```python
from build123d import *

# Parameters (mm, degrees)
CROQUIS1_R                   = 5.25
SALIENTE_EXTRUIR1_DEPTH      = 10
CROQUIS2_R                   = 3
CORTAR_EXTRUIR1_DEPTH        = 10
SALIENTE_EXTRUIR2_DEPTH      = 2
SALIENTE_EXTRUIR2_DEPTH_BACK = 10
CROQUIS3_R                   = 1.25
REDONDEO1_R                  = 1.25


with BuildPart() as part:
    # Croquis1 → Saliente-Extruir1 (new body)
    with BuildSketch(Plane(origin=(0, 0, 0), x_dir=(1, 0, 0), z_dir=(0, 1, 0))):
        with Locations(Location((0, 0, 0), (0, 0, 270))):
            Circle(CROQUIS1_R)
    extrude(amount=SALIENTE_EXTRUIR1_DEPTH)

    # Croquis2 → Cortar-Extruir1 (cut)
    with BuildSketch(Plane(origin=(0, 10, 0), x_dir=(1, 0, 0), z_dir=(0, 1, 0))):
        with Locations(Location((0, 0, 0), (0, 0, 270))):
            Circle(CROQUIS2_R)
    extrude(amount=-CORTAR_EXTRUIR1_DEPTH, mode=Mode.SUBTRACT)

    # Croquis3 → Saliente-Extruir2 (add, two sides: drawn at the far end of the back side and taken through both)
    with BuildSketch(Plane(origin=(0, 10, 0), x_dir=(1, 0, 0), z_dir=(0, 1, 0)).offset(-SALIENTE_EXTRUIR2_DEPTH_BACK)):
        with Locations(Location((0, 3, 0), (0, 0, 270))):
            Circle(CROQUIS3_R)
        with Locations(Location((2.599576211, -1.499133975, 0), (0, 0, 270))):
            Circle(CROQUIS3_R)
        with Locations(Location((-2.596576211, -1.500866025, 0), (0, 0, 270))):
            Circle(CROQUIS3_R)
    extrude(amount=SALIENTE_EXTRUIR2_DEPTH + SALIENTE_EXTRUIR2_DEPTH_BACK)

    # Redondeo1
    redondeo1_edges = [part.edges().sort_by_distance(p)[0] for p in [
        (0, 12, -4.25),
        (2.599576211, 12, 0.249133975),
        (-2.596576211, 12, 0.250866025),
    ]]
    fillet(redondeo1_edges, radius=REDONDEO1_R)


solid = part.part
```
The model under review builds one solid part; all positions refer to its coordinate system, in mm. Round coordinates to 2 decimals unless told otherwise and drop trailing zeros. Loops run counter-clockwise (first coordinate to the right, second up) from the corner with the lowest first, then second, coordinate; pieces in that order, holes last. Notation, with made-up numbers: (11, -34) - (42, -34) arc R28 ccw to (42, -5) - close; hole circle Ø11 at (-20.75, -27). An arc over 180 degrees is marked (long way). Use a Markdown table: item, result. Add a question column.
Q1. Insertion check: pin 1 Ø2 at (x, y) = (4, 4.5) entering from +Z; pin 2 Ø2 at (y, z) = (10, 2) entering from +X; pin 3 Ø4 at (y, z) = (5.5, -4) entering from -X. Each pin has a flat end and moves straight along its axis. Give the tip position at first contact, or say it passes through.
Q2. Add section A-A (x = 0). State the section outline as (y, z) points.
Q3. The part is to be moulded in two halves that separate along Z. For faces 1 (the face through (-2.6, 5.1, -1.5)), 2 (the face through (-2, 0, 1)), 3 (the face through (1.6, 4.9, 5)), say which applies: pulls with the +Z half, pulls with the -Z half, needs draft (parallel to the pull), parting line crosses it, or undercut.
Q4. For probe 1 along Z at (x, y) = (-1.5, 1.25); probe 2 along Y at (x, z) = (3.5, 3.25); probe 3 along X at (y, z) = (8.25, -2), list the stretches that pass through material, from the lowest coordinate up.
Q5. Add section D-D (x = -1.5). State the section outline as (y, z) points, plus the area to 3 significant figures.
Q6. Add section B-B (z = 0). State the section outline as (x, y) points, plus the area to 3 significant figures.
Q7. Add section C-C (y = 6.75). State the section outline as (x, z) points.
Worked answers:
| question | item | result |
|---|---|---|
| 1 | pin 1 | z = 4.31 |
| 1 | pin 2 | x = 5.15 |
| 1 | pin 3 | x = -4.85 |
| 2 | outline | (0, -5.25) - (10, -5.25) - (10, -4.25) - (10.75, -4.25) arc R1.25 ccw to (10.75, -1.75) - (0, -1.75) - close; (0, 3) - (10, 3) - (10, 5.25) - (0, 5.25) - close |
| 3 | face 1 | undercut |
| 3 | face 2 | needs draft |
| 3 | face 3 | parting line crosses it |
| 4 | probe 1 | -5.03 to -2.6, 0.9 to 2.1, 2.6 to 5.03 |
| 4 | probe 2 | 0 to 10 |
| 4 | probe 3 | -4.85 to -2.24, -0.75 to 0.75, 2.24 to 4.85 |
| 5 | outline | (0, -5.03) - (10, -5.03) - (10, -2.6) - (0, -2.6) - close; (0, 0.9) - (10.75, 0.9) arc R0.6 ccw to (10.75, 2.1) - (0, 2.1) - close; (0, 2.6) - (10, 2.6) - (10, 5.03) - (0, 5.03) - close |
| 5 | area | 62.1 mm² |
| 6 | outline | (-5.25, 0) - (-3, 0) - (-3, 10) - (-5.25, 10) - close; (3, 0) - (5.25, 0) - (5.25, 10) - (3, 10) - close |
| 6 | area | 45.0 mm² |
| 7 | outline | circle Ø10.5 at (0, 0); hole (-2.98, 0.31) arc R3 ccw to (-1.22, -2.74) arc R1.25 cw to (1.22, -2.74) arc R3 ccw to (2.98, 0.31) arc R1.25 cw to (1.76, 2.43) arc R3 ccw to (-1.76, 2.43) arc R1.25 cw to start |
